For this review, take the finished solid that the model builds, in its own axes (mm). A direction names the side the tool comes from. Coordinates: 2 decimals unless noted, no trailing zeros. Order: outer loops, then holes, each group sorted by start corner. A loop starts at its lowest first (then second) coordinate and runs counter-clockwise, first axis right, second up. Notation, with made-up numbers: (-22, 74) -> (3, 74) arc R22 cw to (3, 113) -> close; hole circle Ø11 at (-35, 80). An arc over 180 degrees is marked (long way). Answer as a JSON object with one key per item and string values. Group by question number.
1) Add section C-C, the plane y = -36. Write out the cut boundary in (x, z).
2) Wall thickness on L1, parallel to X at y = -20.5, z = -8.5; L2, parallel to X at y = -7.5, z = -3; L3, parallel to X at y = -11, z = -6: over which ranges is each line inside the solid? List them lowest first.
3) Add section D-D, the plane z = -2.75. Write out the cut boundary in (x, y).
4) Add section A-A, the plane z = -8.75. Write out the cut boundary in (x, y).
5) Machinability: for faces 1 (the cylindrical face through (-7.45, -38.77, -2.25)), 2 (the cylindrical face through (7.6, -31.4, -4)), which of the approach directions +Z, -Z, +X, -X, +Y, -Y give a long, thin tool a straight path to every point of the face, cutting with its end or side? Answer none if there is none.
6) Add section B-B, the plane x = 7.5. Write out the cut boundary in (y, z), then the cut area to 3 significant figures.
7) For pin 1 (4 mm diameter, centred on x = -9, y = -5.5, fed in from +Z), flat-tipped, find the tip position at first contact; note if it passes through.
8) Draft analysis for pull direction X (two halves, no side actions). For faces 3 (the flat face through (4, -20, -9)), 4 (the flat face through (15, -20, -5)), 5 (the flat face through (-13, -20, 0)), state which applies: +X half, -X half, draft (parallel to the pull), parting line (faces both ways), or undercut.
from build123d import *

# Parameters (mm, degrees)
SKETCH_1_W               = 30
SKETCH_1_H               = 10
EXTRUDE_1_DEPTH          = 40
CUT_EXTRUDE_START        = -1.5
SKETCH_2_R               = 4
CUT_EXTRUDE_1_DEPTH      = 12
CUT_EXTRUDE_START_2      = -12
CUT_EXTRUDE_2_DEPTH      = 12
CUT_EXTRUDE_3_DEPTH      = 33.050741021
CUT_EXTRUDE_3_DEPTH_BACK = 33.050741021
SKETCH_4_R               = 2.25
CUT_EXTRUDE_4_DEPTH      = 44.874821937


with BuildPart() as part:
    # 草图1 → 凸台-拉伸1 (new body)
    with BuildSketch(Plane(origin=(0, 0, 0), x_dir=(1, 0, 0), z_dir=(0, 1, 0))):
        with Locations((0, 5)):
            Rectangle(SKETCH_1_W, SKETCH_1_H)
    extrude(amount=-EXTRUDE_1_DEPTH)

    # 草图2 → 切除-拉伸1 (cut)
    with BuildSketch(Plane(origin=(0, 0, 0), x_dir=(1, 0, 0), z_dir=(0, 1, 0)).offset(CUT_EXTRUDE_START)):
        with Locations((-7.5, 0)):
            Circle(SKETCH_2_R)
        with Locations((7.5, 0)):
            Circle(SKETCH_2_R)
    extrude(amount=-CUT_EXTRUDE_1_DEPTH, mode=Mode.SUBTRACT)

    # 草图3 → 切除-拉伸2 (cut)
    with BuildSketch(Plane(origin=(0, -13.5, 0), x_dir=(1, 0, 0), z_dir=(0, 1, 0)).offset(CUT_EXTRUDE_START_2)):
        with BuildLine():
            Line((-11.5, 0), (-3.5, 0))
            ThreePointArc((-3.5, 0), (-7.5, 4), (-11.5, 0))
        make_face()
        with BuildLine():
            Line((3.5, 0), (11.5, 0))
            ThreePointArc((11.5, 0), (7.5, 4), (3.5, 0))
        make_face()
    extrude(amount=-CUT_EXTRUDE_2_DEPTH, mode=Mode.SUBTRACT)

    # 草图4 → 切除-拉伸3 (cut, two sides: drawn at the far end of the back side and taken through both)
    with BuildSketch(Plane(origin=(0, -13.5, 0), x_dir=(1, 0, 0), z_dir=(0, 1, 0)).offset(-CUT_EXTRUDE_3_DEPTH_BACK)):
        with Locations((-7.5, 0)):
            Circle(SKETCH_4_R)
        with Locations((7.5, 0)):
            Circle(SKETCH_4_R)
    extrude(amount=CUT_EXTRUDE_3_DEPTH + CUT_EXTRUDE_3_DEPTH_BACK, mode=Mode.SUBTRACT)

    # 草图5 → 切除-拉伸4 (cut, through all)
    with BuildSketch(Plane(origin=(0, 0, 0), x_dir=(1, 0, 0), z_dir=(0, 1, 0))):
        with BuildLine():
            Line((-4, 7.5), (-4, 10))
            ThreePointArc((-4, 10), (0, 14), (4, 10))
            Line((4, 10), (4, 7.5))
            ThreePointArc((4, 7.5), (0, 3.5), (-4, 7.5))
        make_face()
    extrude(amount=-CUT_EXTRUDE_4_DEPTH, mode=Mode.SUBTRACT)


solid = part.part
Output values:
{
 "1": {"outline": "(-15, -10) -> (-4, -10) -> (-4, -7.5) arc R4 cw to (4, -7.5) -> (4, -10) -> (15, -10) -> (15, 0) -> (11.5, 0) arc R4 cw to (3.5, 0) -> (-3.5, 0) arc R4 cw to (-11.5, 0) -> (-15, 0) -> close"},
 "2": {"L1": "x = -15 to -4, 4 to 15", "L2": "x = -15 to -10.15, -4.85 to 4.85, 10.15 to 15", "L3": "x = -15 to -3.71, 3.71 to 15"},
 "3": {"outline": "(-15, -40) -> (15, -40) -> (15, 0) -> (-15, 0) -> close; hole (-10.4, -37.5) -> (-4.6, -37.5) -> (-4.6, -25.5) -> (-10.4, -25.5) -> close; hole (-10.4, -13.5) -> (-4.6, -13.5) -> (-4.6, -1.5) -> (-10.4, -1.5) -> close; hole (4.6, -37.5) -> (10.4, -37.5) -> (10.4, -25.5) -> (4.6, -25.5) -> close; hole (4.6, -13.5) -> (10.4, -13.5) -> (10.4, -1.5) -> (4.6, -1.5) -> close"},
 "4": {"outline": "(-15, -40) -> (-4, -40) -> (-4, 0) -> (-15, 0) -> close; (4, -40) -> (15, -40) -> (15, 0) -> (4, 0) -> close"},
 "5": {"face 1": "+Z, +Y, -Y", "face 2": "+Z"},
 "6": {"outline": "(-40, -10) -> (0, -10) -> (0, -2.25) -> (-1.5, -2.25) -> (-1.5, -4) -> (-13.5, -4) -> (-13.5, -2.25) -> (-25.5, -2.25) -> (-25.5, -4) -> (-37.5, -4) -> (-37.5, -2.25) -> (-40, -2.25) -> close", "area": "268 mm²"},
 "7": {"pin 1": "stops at z = -1.94"},
 "8": {"face 3": "undercut", "face 4": "+X half", "face 5": "draft"}
}
